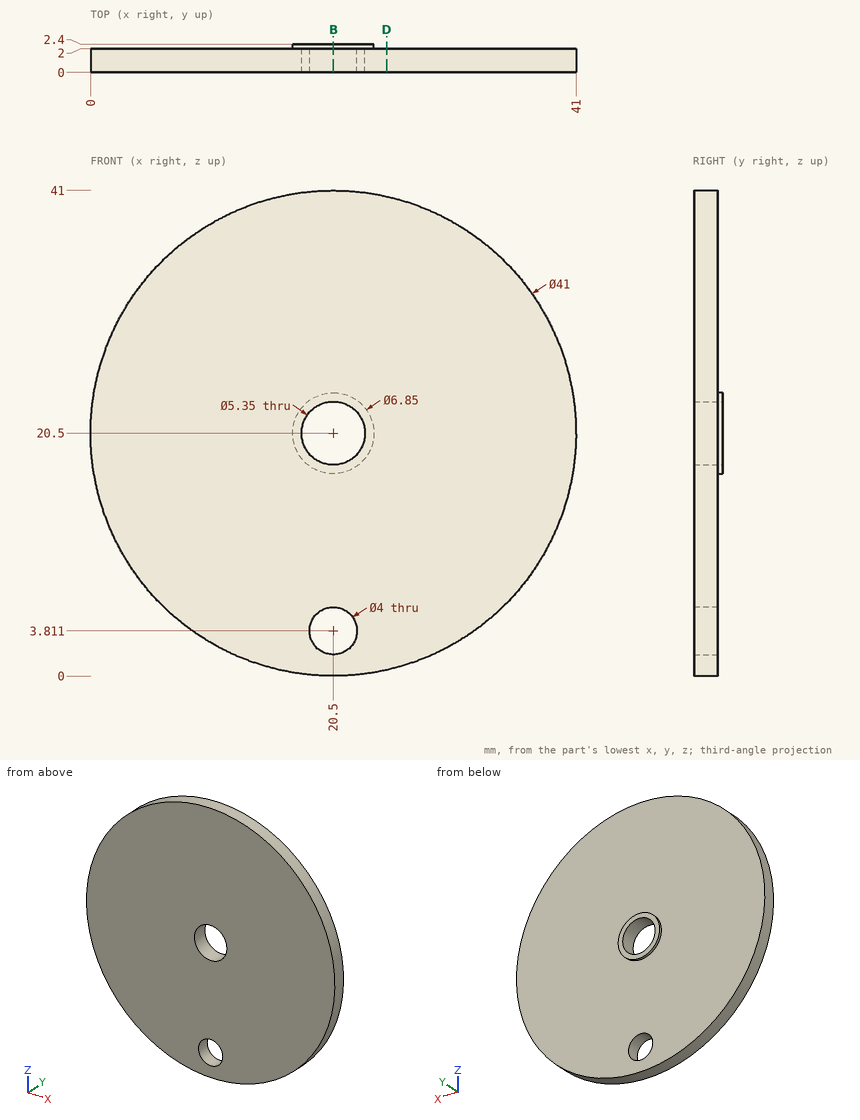
Here's the drawing with two shaded views (mm, measured from the low corner). I have some questions. Coordinates: 2 decimals unless noted, no trailing zeros. Order: outer loops, then holes, each group sorted by start corner. A loop starts at its lowest first (then second) coordinate and runs counter-clockwise, first axis right, second up.
Q1. Will these pins go through, and if not, where does the flat tip stop? pin 1 (2 mm diameter, centred on x = 9.5, z = 18.5, fed in from +Y); pin 2 (5 mm diameter, centred on x = 20.5, z = 20.5, fed in from -Y); pin 3 (1 mm diameter, centred on y = 2, z = 30, fed in from -X); pin 4 (1 mm diameter, centred on x = 7.5, y = 1.5, fed in from +Z).
Q2. Please list where these lines run through material, in increasing order: L1, parallel to Z at x = 21, y = 0.25 (1 decimal); L2, parallel to X at y = 1.5, z = 20.5 (1 decimal); L3, parallel to Y at x = 19, z = 13.
Q3. Suppose I cut it at B-B on x = 20.5. Give the number of separate pieces and of enclosed holes in the cut face.
Q4. Suppose I cut it at D-D on x = 25. Please give me the cut outline in (y, z).
Answer:
1. pin 1: stops at y = 2
1. pin 2: passes through
1. pin 3: stops at x = 2.08
1. pin 4: stops at z = 36.75
2. L1: z = 0 to 1.9, 5.7 to 17.9, 23.1 to 41
2. L2: x = 0 to 17.8, 23.2 to 41
2. L3: y = 0 to 2
3. separate pieces: 3
3. enclosed holes: 0
4. outline: (0, 0.5) - (2, 0.5) - (2, 40.5) - (0, 40.5) - close
